For this review, use the dimensioned drawing (mm, ordinates from the lowest corner) and the shaded views. A direction names the side the tool comes from. Give positions to 0.01 mm unless a question says otherwise; leave off trailing zeros. Write each loop counter-clockwise with the first axis right and the second up, starting at its lowest first coordinate (ties: lowest second). Pieces come first, ordered by that corner, then holes. Notation, with made-up numbers: M -1,7 L 37,7 A9 cw 37,19 Z; hole C 62,-36.75 d7. An arc over 180 degrees is marked long. Answer in a Markdown table with one row per item.
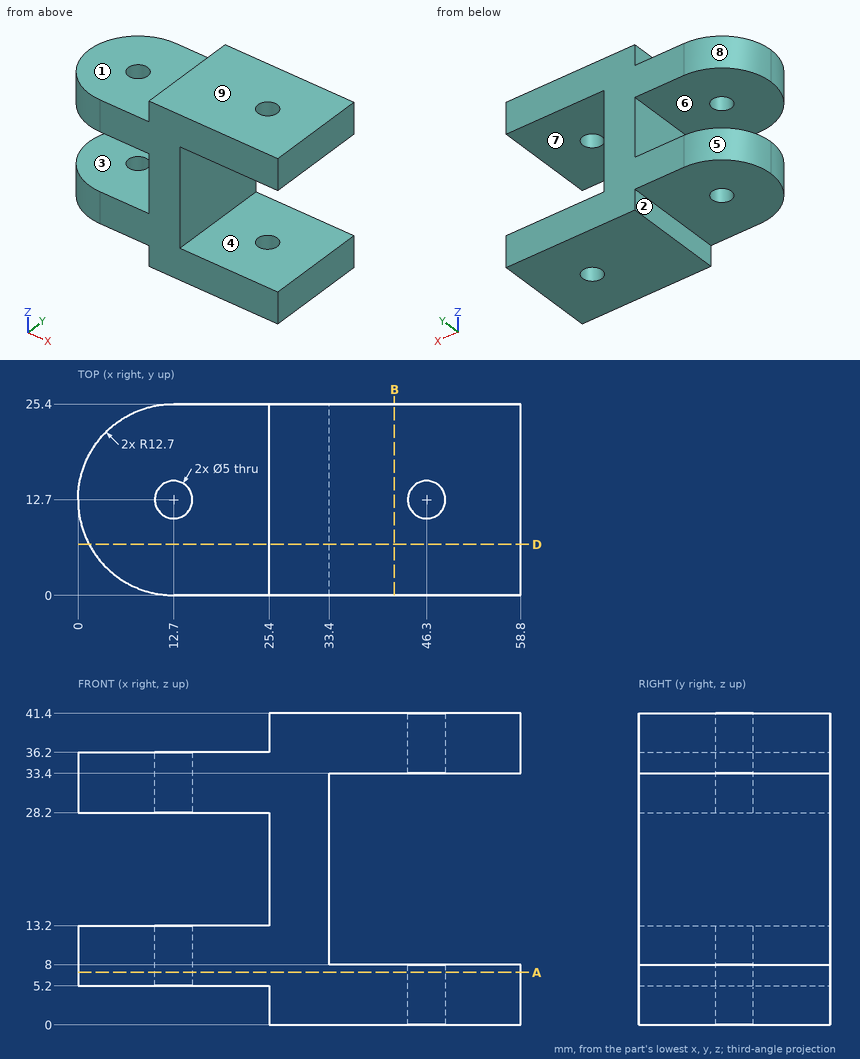
1) Add section B-B (x = 42). Write out the cut boundary in (y, z).
Geometry says:
| item | result |
|---|---|
| outline | M 0,0 L 25.4,0 L 25.4,8 L 0,8 Z; M 0,33.4 L 25.4,33.4 L 25.4,41.4 L 0,41.4 Z |
2) Insertion check: P1, Ø4.5, axis at y = 7.5, z = 22, coming from the -X side; P2, Ø12.5, axis at x = 10.5, y = 7.5, coming from the +Z side; P3, Ø6, axis at y = 14.5, z = 12, coming from the +X side. Each pin has a flat end and moves straight along its axis. Give the tip position at first contact, or say it passes through.
Geometry says:
| item | result |
|---|---|
| P1 | x = 25.4 |
| P2 | z = 36.2 |
| P3 | x = 33.4 |
3) For the marked faces 1, 2, 3, 4 and 5, list the 3-axis set-ups (+Z, -Z, +X, -X, +Y, -Y) from which the entire face can be reached by the end or side of a thin tool; tool diameter is ignored.
Geometry says:
| item | result |
|---|---|
| face 1 | +Z, -X, +Y, -Y |
| face 2 | -Z, -X, +Y, -Y |
| face 3 | -X, +Y, -Y |
| face 4 | +X, +Y, -Y |
| face 5 | +Z, -Z, -X, +Y |
4) Add section D-D (y = 6.75). Write out the cut boundary in (x, z).
Geometry says:
| item | result |
|---|---|
| outline | M 1.48,5.2 L 25.4,5.2 L 25.4,0 L 58.8,0 L 58.8,8 L 33.4,8 L 33.4,33.4 L 58.8,33.4 L 58.8,41.4 L 25.4,41.4 L 25.4,36.2 L 1.48,36.2 L 1.48,28.2 L 25.4,28.2 L 25.4,13.2 L 1.48,13.2 Z |
5) To check wall thickness, follow probe 1 along Z at (x, y) = (44, 23); probe 2 along Y at (x, z) = (12.7, 7.25); probe 3 along Z at (x, y) = (8.5, 2.5). State the ranges of each line that lie inside material, in increasing order. Write a range as [from, to].
Geometry says:
| item | result |
|---|---|
| probe 1 | [0, 8], [33.4, 41.4] |
| probe 2 | [0, 10.2], [15.2, 25.4] |
| probe 3 | [5.2, 13.2], [28.2, 36.2] |
6) The part is to be moulded in two halves that separate along Z. For the marked faces 6, 7, 8 and 9, say which applies: released by +Z, released by -Z, zero draft, split by the parting line, or undercut.
Geometry says:
| item | result |
|---|---|
| face 6 | undercut |
| face 7 | undercut |
| face 8 | zero draft |
| face 9 | released by +Z |
7) Add section A-A (z = 7). Count the separate pieces of the cut face and the enclosed holes in it, and give its area (4 significant figures).
Geometry says:
| item | result |
|---|---|
| separate pieces | 1 |
| enclosed holes | 2 |
| area | 1,385 mm^2 |
